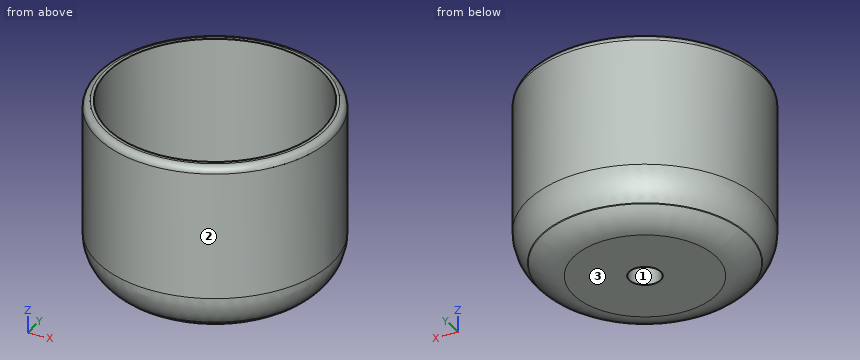
from build123d import *

# Parameters (mm, degrees)
F0_R     = 13
F1_DEPTH = 20
F2_R     = 11.9
F3_DEPTH = 17
F4_R     = 1.75
F5_DEPTH = 4.1
F6_SIZE  = 3
F7_R     = 5
F8_R     = 0.75


with BuildPart() as f1:
    # F0 (on Top) → F1 (new body)
    with BuildSketch(Plane.XY):
        Circle(F0_R)
    extrude(amount=F1_DEPTH)

    # F2 (on face) → F3 (cut)
    with BuildSketch(Plane.XY.offset(20)):
        Circle(F2_R)
    extrude(amount=-F3_DEPTH, mode=Mode.SUBTRACT)

    # F4 (on Top) → F5 (cut)
    with BuildSketch(Plane.XY):
        Circle(F4_R)
    extrude(amount=F5_DEPTH, mode=Mode.SUBTRACT)

    # F6
    f6_edges = [f1.edges().sort_by_distance(p)[0] for p in [
        (-13, 0, 0),
    ]]
    chamfer(f6_edges, length=F6_SIZE)

    # F7
    f7_edges = [f1.edges().sort_by_distance(p)[0] for p in [
        (-10, 0, 0),
        (-13, 0, 3),
    ]]
    fillet(f7_edges, radius=F7_R)

    # F8
    f8_edges = [f1.edges().sort_by_distance(p)[0] for p in [
        (-13, 0, 20),
    ]]
    fillet(f8_edges, radius=F8_R)


solid = f1.part
The model under review builds one solid part; all positions refer to its coordinate system, in mm. Face numbers are marked on the shaded views. Round coordinates to 2 decimals unless told otherwise and drop trailing zeros. Write each loop counter-clockwise with the first axis right and the second up, starting at its lowest first coordinate (ties: lowest second). Pieces come first, ordered by that corner, then holes. Notation, with made-up numbers: (89, -12) - (108, -12) arc R21 ccw to (108, 9) - close; hole circle Ø11 at (-24, 49). An arc over 180 degrees is marked (long way). One line per item, written item: value. Start each with the question number.
1. To check wall thickness, follow L1, parallel to Y at x = 0, z = 12.25; L2, parallel to Y at x = -2.25, z = 18.5; L3, parallel to Z at x = -3.75, y = -0.75. State the ranges of each line that lie inside material, in increasing order. Write a range as from..to.
2. Consider section A-A on z = 18.75. Write out the cut boundary in (x, y), and give its area (3 significant figures).
3. Clearance check with flat-ended pins moving along their axes: P1, Ø5, axis at y = -6, z = 17, coming from the -X side; P2, Ø4, axis at x = -3, z = 6.5, coming from the +Y side; P3, Ø12, axis at x = -9.5, y = 4.5, coming from the -Z side; P4, Ø6, axis at x = 6.5, z = 13.5, coming from the +Y side. State where each tip first meets the part, or that it passes through.
4. The part is to be moulded in two halves that separate along X. For the marked faces 1, 2 and 3, say which applies: released by +X, released by -X, zero draft, split by the parting line, or undercut.
Checks:
1. L1: y = -13..-11.9, 11.9..13
1. L2: y = -12.8..-11.69, 11.69..12.8
1. L3: z = 0..3
2. outline: circle Ø26 at (0, 0); hole circle Ø23.8 at (0, 0)
2. area: 86.0 mm^2
3. P1: stops at x = -12.52
3. P2: stops at y = 12.96
3. P3: stops at z = 0
3. P4: stops at y = 12.52
4. face 1: undercut
4. face 2: split by the parting line
4. face 3: zero draft
